Model file for the job. Use its own axes, mm. Face numbers are marked on the shaded views. A direction names the side the tool comes from. Coordinates: 2 decimals unless noted, no trailing zeros. Order: outer loops, then holes, each group sorted by start corner. A loop starts at its lowest first (then second) coordinate and runs counter-clockwise, first axis right, second up.
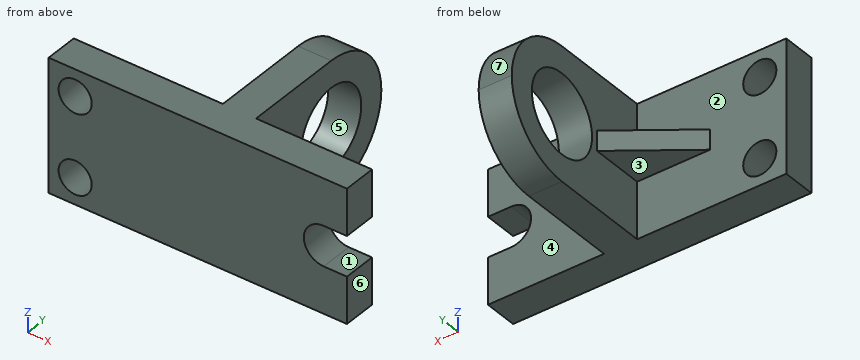
from build123d import *

# Parameters (mm, degrees)
EXTRUDE_1_DEPTH      = 10
EXTRUDE_1_DEPTH_BACK = 10
SKETCH_1_W           = 40
SKETCH_1_H           = 5
EXTRUDE_2_DEPTH      = 1.5
EXTRUDE_2_DEPTH_BACK = 1.5
FILLET_1_R           = 10
SKETCH_2_R           = 6
CUT_EXTRUDE_1_DEPTH  = 37.912057651
SKETCH_4_R           = 3
CUT_EXTRUDE_3_DEPTH  = 34.541019662
SKETCH_5_W           = 20
SKETCH_5_H           = 5
EXTRUDE_3_DEPTH      = 5
SKETCH_3_R           = 2.5
CUT_EXTRUDE_4_DEPTH  = 37.742346142


with BuildPart() as part:
    # Эскиз1 → Бобышка-Вытянуть1 (new, two sides: drawn at the far end of the back side and taken through both)
    with BuildSketch(Plane.XY.offset(-EXTRUDE_1_DEPTH_BACK)):
        Rectangle(SKETCH_1_W, SKETCH_1_H)
        Polygon((-2.5, 27.5), (-2.5, 10.5), (-2.5, 2.5), (2.5, 2.5), (2.5, 27.5), align=None)
    extrude(amount=EXTRUDE_1_DEPTH + EXTRUDE_1_DEPTH_BACK)

    # Эскиз1<3> → Бобышка-Вытянуть2 (add, two sides: drawn at the far end of the back side and taken through both)
    with BuildSketch(Plane.XY.offset(-EXTRUDE_2_DEPTH_BACK)):
        Polygon((-2.5, 10.5), (-13.5, 2.5), (-2.5, 2.5), align=None)
    extrude(amount=EXTRUDE_2_DEPTH + EXTRUDE_2_DEPTH_BACK)

    # Скругление1
    fillet_1_edges = [part.edges().sort_by_distance(p)[0] for p in [
        (0, 27.5, 10),
        (0, 27.5, -10),
    ]]
    fillet(fillet_1_edges, radius=FILLET_1_R - 0.0001)  # a hair under: the kernel refuses the full size

    # Эскиз2 → Вырез-Вытянуть1 (cut, through all)
    with BuildSketch(Plane.ZY.offset(2.5)):
        with Locations(Location((0, 17.5, 0), (0, 0, 270))):
            Circle(SKETCH_2_R)
    extrude(amount=-CUT_EXTRUDE_1_DEPTH, mode=Mode.SUBTRACT)

    # Эскиз4 → Вырез-Вытянуть3 (cut, through all)
    with BuildSketch(Plane(origin=(0, 2.5, 0), x_dir=(1, 0, 0), z_dir=(0, 1, 0))):
        with BuildLine():
            Line((20, 3), (16.5, 3))
            ThreePointArc((16.5, 3), (18.621320344, 2.121320344), (19.5, 0))
            ThreePointArc((19.5, 0), (18.621320344, -2.121320344), (16.5, -3))
            Line((16.5, -3), (20, -3))
            Line((20, -3), (20, 3))
        make_face()
        with Locations((16.5, 0)):
            Circle(SKETCH_4_R)
    extrude(amount=-CUT_EXTRUDE_3_DEPTH, mode=Mode.SUBTRACT)

    # Эскиз5 → Бобышка-Вытянуть3 (add)
    with BuildSketch(Plane.ZY.offset(20)):
        Rectangle(SKETCH_5_W, SKETCH_5_H)
    extrude(amount=EXTRUDE_3_DEPTH)

    # Эскиз3 → Вырез-Вытянуть4 (cut, through all)
    with BuildSketch(Plane(origin=(0, 2.5, 0), x_dir=(1, 0, 0), z_dir=(0, 1, 0))):
        with Locations(Location((-21, -6, 0), (0, 0, 270))):
            Circle(SKETCH_3_R)
    cut_extrude_4 = extrude(amount=-CUT_EXTRUDE_4_DEPTH, mode=Mode.SUBTRACT)

    # Зеркальное отражение1: Вырез-Вытянуть4 across plane
    add(cut_extrude_4.mirror(Plane.XY), mode=Mode.SUBTRACT)


solid = part.part
Q1. Cut at B-B, the plane x = -21. List the corners of the cut face in (y, z).
Established:
outline: (-2.5, -10) - (2.5, -10) - (2.5, -8.5) - (-2.5, -8.5) - close; (-2.5, -3.5) - (2.5, -3.5) - (2.5, 3.5) - (-2.5, 3.5) - close; (-2.5, 8.5) - (2.5, 8.5) - (2.5, 10) - (-2.5, 10) - close
Q2. Probe line 1 (X direction, y = -0.4, z = -6); line 2 (Y direction, x = -5, z = -3). List the from-to ranges inside material, lowest first.
Established:
line 1: x = -25 to -23.5, -18.5 to 20
line 2: y = -2.5 to 2.5
Q3. Cut at C-C, the plane z = 0.75. List the corners of the cut face in (x, y), plus the area to 3 significant figures.
Established:
outline: (-25, -2.5) - (13.6, -2.5) - (13.6, 2.5) - (2.5, 2.5) - (2.5, 11.55) - (-2.5, 11.55) - (-2.5, 10.5) - (-13.5, 2.5) - (-25, 2.5) - close; (-2.5, 23.45) - (2.5, 23.45) - (2.5, 27.47) - (-2.5, 27.47) - close
area: 302 mm2
Q4. Mould opens along Y. For the marked faces 5, 6 and 7 say: pulls with the +Y half, pulls with the -Y half, needs draft (parallel to the pull), parting line crosses it, or undercut.
Established:
face 5: undercut
face 6: needs draft
face 7: pulls with the +Y half
Q5. Cut at D-D, the plane y = 17. List the corners of the cut face in (x, z), plus the area to 3 significant figures.
Established:
outline: (-2.5, -10) - (2.5, -10) - (2.5, -5.98) - (-2.5, -5.98) - close; (-2.5, 5.98) - (2.5, 5.98) - (2.5, 10) - (-2.5, 10) - close
area: 40.2 mm2
Q6. Drop flat-ended pins along their axis: P1, Ø8, axis at x = -9, z = 4, coming from the +Y side; P2, Ø3, axis at x = -21, z = 6, coming from the +Y side; P3, Ø10, axis at y = 17, z = -2, coming from the -X side; P4, Ø9, axis at x = -6, y = 5, coming from the +Z side. Give the stop position or say it passes through.
Established:
P1: stops at y = 8.04
P2: passes through
P3: stops at x = -2.5
P4: stops at z = 10
Q7. Which spindle directions (+Z, -Z, +X, -X, +Y, -Y) get a long thin tool onto all of the face, cutting with end or side? Do the marked faces 1, 2, 3 and 4. Say none if no direction does.
Established:
face 1: +X, +Y, -Y
face 2: -X, +Y
face 3: -Z, -X, +Y
face 4: +Z, -Z, +X, +Y
